from build123d import *

# Parameters (mm, degrees)
F3_W     = 421.7902910393
F3_H     = 198.2180179606
F4_DEPTH = 25.4


# Not quite as in the source:
# - ends of sketch curves that miss each other by under 0.0002 mm in the source are joined


with BuildPart() as f1:
    # F0 (on Front) → F1 (revolve)
    with BuildSketch(Plane.XZ):
        with BuildLine():
            Line((10.5788812285, 8.2366884696), (-24.2557799278, 8.2366884696))
            Line((-24.2557799278, 8.2366884696), (-24.6392214836, 8.2366884696))
            ThreePointArc((-24.6392214836, 8.2366884696), (-32.6864160689, -0.0082121834), (-24.6228011914, -8.2370543))
            Line((-24.6228011914, -8.2370543), (-24.27220022, -8.2370543))
            Line((-24.27220022, -8.2370543), (10.5788812285, -8.2370543))
            Line((10.5788812285, -8.2370543), (10.5788812285, 8.2366884696))
        make_face()
    revolve(axis=Axis((10.5788812285, 0, -0.0001829152), (0, 0, -1)))

    # F3 (on offset) → F4 (cut)
    with BuildSketch(Plane.XY.offset(10)):
        Rectangle(F3_W, F3_H)
        with BuildLine():
            ThreePointArc((-10.7153009133, 20.1523680538), (-0.8347905086, 26.6913979084), (10.7887436299, 28.9885377447))
            ThreePointArc((10.7887436299, 28.9885377447), (22.3773621495, 26.6792950108), (32.203329708, 20.1158334422))
            ThreePointArc((32.203329708, 20.1158334422), (38.769051111, 10.2908037813), (41.0760354322, -1.2987526262))
            ThreePointArc((41.0760354322, -1.2987526262), (38.7450627408, -12.8738402066), (32.1768729102, -22.6858234277))
            ThreePointArc((32.1768729102, -22.6858234277), (22.3718072579, -29.2722876696), (10.7887436292, -31.5860449158))
            ThreePointArc((10.7887436292, -31.5860449158), (-0.8256146846, -29.2802975648), (-10.6861755573, -22.7244524913))
            ThreePointArc((-10.6861755573, -22.7244524913), (-17.3142524075, -12.9103633574), (-19.6419716109, -1.2987526263))
            ThreePointArc((-19.6419716109, -1.2987526263), (-17.3228833961, 10.3191134223), (-10.7153009133, 20.1523680538))
        make_face(mode=Mode.SUBTRACT)
    extrude(amount=-F4_DEPTH, mode=Mode.SUBTRACT)


solid = f1.part
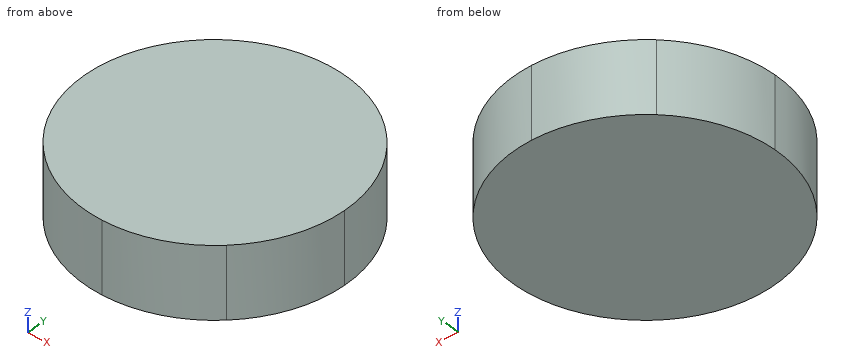
Model file for the job. Use its own axes, mm. Give positions to 0.01 mm unless a question says otherwise; leave off trailing zeros. Order: outer loops, then holes, each group sorted by start corner. A loop starts at its lowest first (then second) coordinate and runs counter-clockwise, first axis right, second up. Notation, with made-up numbers: (32, -1) - (52, -1) arc R31 cw to (52, 24) - close; hole circle Ø6 at (79.25, 88). An arc over 180 degrees is marked (long way). One line per item, written item: value.
Item 1: Pin check, flat tips, straight feed: pin 1 Ø8 at (x, z) = (35, 2) entering from -Y; pin 2 Ø2 at (y, z) = (8, 4.5) entering from +X; pin 3 Ø2 at (y, z) = (-22, -0.5) entering from -X. Stop position of each tip, or through.
Response values:
pin 1: y = -23.81
pin 2: x = 39.92
pin 3: x = -12.3
Item 2: Slice it at B-B (x = 35). List the corners of the cut face in (y, z), then the cut area to 3 significant figures.
Response values:
outline: (-19.43, -8.24) - (16.89, -8.24) - (16.89, 8.24) - (-19.43, 8.24) - close
area: 598 mm2
Item 3: Wall check: line 1 (Y direction, x = 12.5, z = -2.25); line 2 (Y direction, x = 16, z = -1.75); line 3 (X direction, y = 11, z = 5.25). Give the ranges that are in metal, low to high.
Response values:
line 1: -31.54 to 28.94
line 2: -31.13 to 28.53
line 3: -17.03 to 38.46
Item 4: Slice it at A-A (z = 5.25). List the corners of the cut face in (x, y), then the cut area to 3 significant figures.
Response values:
outline: (-19.64, -1.3) arc R30.09 ccw to (-10.69, -22.72) arc R30.5 ccw to (10.79, -31.59) arc R30.15 ccw to (32.18, -22.69) arc R30.38 ccw to (41.08, -1.3) arc R30.29 ccw to (32.2, 20.12) arc R30.32 ccw to (10.79, 28.99) arc R30.61 ccw to (-10.72, 20.15) arc R30.22 ccw to start
area: 2,890 mm2
Item 5: Slice it at C-C (y = -7.5). List the corners of the cut face in (x, z), then the cut area to 3 significant figures.
Response values:
outline: (-19, -8.24) - (40.42, -8.24) - (40.42, 8.24) - (-19, 8.24) - close
area: 979 mm2
